from build123d import *

# Parameters (mm, degrees)
F1_DEPTH    = 6.35
F2_T1_DEPTH = 12.8820747894
F2_T3_DEPTH = 11.6021811914
F4_D        = 10.0838
F6_D        = 5.1054


# Not quite as in the source:
# - a fillet or chamfer that OpenCascade refuses, or shapes differently, is made with other operations: its cross-section is extruded or revolved along the edge and cut away or added


with BuildPart() as f1:
    # F0 (on Front) → F1 (new body)
    with BuildSketch(Plane.XZ):
        Polygon((0, -38.1), (0, 0), (-215.9, 0), (-215.9, -15.24), (-116.8824615139, -38.1), align=None)
    extrude(amount=-F1_DEPTH)

    # F2: chamfer of 1.27 on 4 edges, made by hand

    # F2_s2 → F2_t1 (cut)
    with BuildSketch(Plane.XZ.offset(-9.6160373947)):
        Polygon((-214.63, 0), (-215.9, -1.27), (-215.9, 0), align=None)
        Polygon((-1.27, -38.1), (0, -36.83), (0, -38.1), align=None)
        Polygon((0, -1.27), (-1.27, 0), (0, 0), align=None)
    extrude(amount=F2_T1_DEPTH, mode=Mode.SUBTRACT)

    # F2_s4 → F2_t3 (cut)
    with BuildSketch(Plane.XZ.offset(-8.9760905957)):
        Polygon((-215.9, -14.2297963858), (-214.915687839, -15.4672463681), (-215.9, -15.24), align=None)
    extrude(amount=F2_T3_DEPTH, mode=Mode.SUBTRACT)

    # F4 (through all)
    with Locations(Plane.XZ):
        with Locations((-50.8, -19.05), (-19.05, -19.05)):
            Hole(F4_D / 2)

    # F6 (through all)
    with Locations(Plane.XZ):
        with Locations((-209.55, -6.35)):
            Hole(F6_D / 2)


solid = f1.part
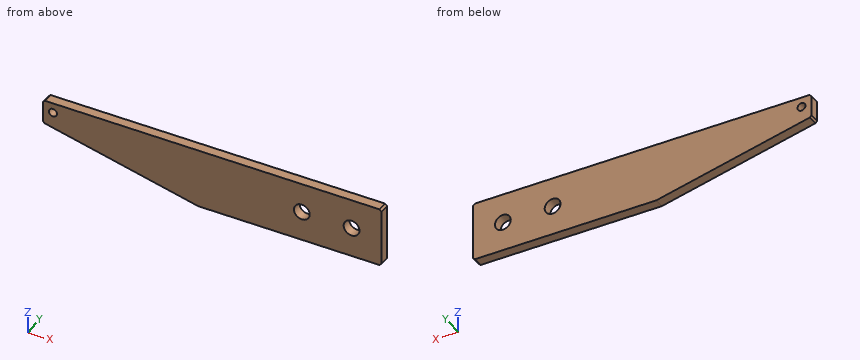
Model file for the job. Use its own axes, mm. Give positions to 0.01 mm unless a question says otherwise; leave off trailing zeros. Write each loop counter-clockwise with the first axis right and the second up, starting at its lowest first coordinate (ties: lowest second). Pieces come first, ordered by that corner, then holes. Notation, with made-up numbers: M 10,69.5 L 38,69.5 A19 cw 38,98.5 Z; hole C 20.5,-15.75 d3. An arc over 180 degrees is marked long. One line per item, written item: value. Start each with the question number.
Q1. Saw through at A-A, the plane x = -50.8. Write the cut outline in (y, z), plus the area to 3 significant figures.
Q2. Saw through at C-C, the plane y = 1.75. Write the cut outline in (x, z), plus the area to 3 significant figures.
Q3. Probe probe 1 along Z at (x, y) = (-51, 2.25); probe 2 along X at (y, z) = (2.5, -15); probe 3 along Z at (x, y) = (-209.55, 2). List the from-to ranges inside material, lowest first. Write a range as [from, to].
Q4. Saw through at D-D, the plane z = -19.05. Write the cut outline in (x, y).
Q5. Drop a flat-ended pin along its axis: pin 1 Ø6 at (x, z) = (-50.8, -19.05) entering from +Y. Give the stop position or say it passes through.
Q6. Saw through at B-B, the plane z = -6.35. Write the cut outline in (x, y).
Output values:
1. outline: M 0,-38.1 L 6.35,-38.1 L 6.35,-24.09 L 0,-24.09 Z; M 0,-14.01 L 6.35,-14.01 L 6.35,0 L 0,0 Z
1. area: 178 mm²
2. outline: M -215.9,-14.23 L -214.92,-15.47 L -116.88,-38.1 L -1.27,-38.1 L 0,-36.83 L 0,-1.27 L -1.27,0 L -214.63,0 L -215.9,-1.27 Z; hole C -209.55,-6.35 d5.11; hole C -50.8,-19.05 d10.08; hole C -19.05,-19.05 d10.08
2. area: 6,910 mm²
3. probe 1: z = [-38.1, -24.09], [-14.01, 0]
3. probe 2: x = [-215.29, -53.8], [-47.8, -22.05], [-16.05, 0]
3. probe 3: z = [-16.71, -8.9], [-3.8, 0]
4. outline: M -199.4,0 L -55.84,0 L -55.84,6.35 L -199.4,6.35 Z; M -45.76,0 L -24.09,0 L -24.09,6.35 L -45.76,6.35 Z; M -14.01,0 L 0,0 L 0,6.35 L -14.01,6.35 Z
5. pin 1: passes through
6. outline: M -215.9,0 L -212.1,0 L -212.1,6.35 L -215.9,6.35 Z; M -207,0 L 0,0 L 0,6.35 L -207,6.35 Z
